from build123d import *

# Parameters (mm, degrees)
SKETCH1_R               = 27.1
SKETCH1_R_2             = 25.2
BOSS_EXTRUDE1_DEPTH     = 300
SKETCH2_R               = 2.9
CUT_EXTRUDE1_DEPTH      = 28.1
CUT_EXTRUDE1_DEPTH_BACK = 28.1


with BuildPart() as part:
    # Sketch1 → Boss-Extrude1 (new body)
    with BuildSketch(Plane(origin=(0, 0, 0), x_dir=(1, 0, 0), z_dir=(0, 1, 0))):
        Circle(SKETCH1_R)
        Circle(SKETCH1_R_2, mode=Mode.SUBTRACT)
    extrude(amount=BOSS_EXTRUDE1_DEPTH)

    # Sketch2 → Cut-Extrude1 (cut, two sides)
    with BuildSketch(Plane(origin=(0, 0, 0), x_dir=(0, 0, -1), z_dir=(1, 0, 0))) as cut_extrude1_sk:
        with Locations((0, 10)):
            Circle(SKETCH2_R)
        with Locations((0, 25.5)):
            Circle(SKETCH2_R)
    extrude(amount=CUT_EXTRUDE1_DEPTH, mode=Mode.SUBTRACT)
    extrude(cut_extrude1_sk.sketch, amount=-CUT_EXTRUDE1_DEPTH_BACK, mode=Mode.SUBTRACT)


solid = part.part
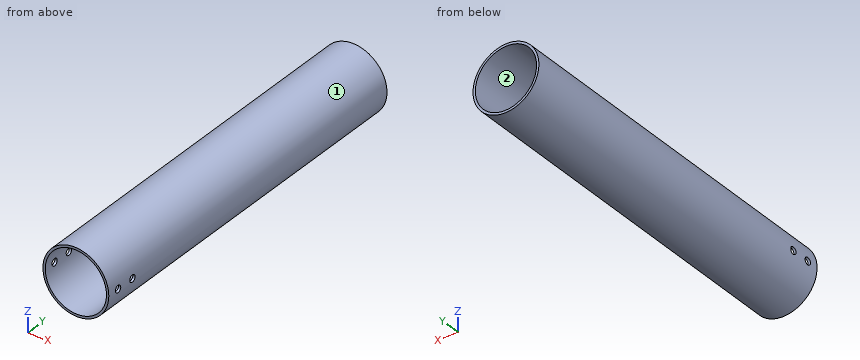
Geometry check sheet. Reference: the model listing, model coordinates, mm. Face numbers are marked on the shaded views. Coordinates: 2 decimals unless noted, no trailing zeros. Order: outer loops, then holes, each group sorted by start corner. A loop starts at its lowest first (then second) coordinate and runs counter-clockwise, first axis right, second up. Notation, with made-up numbers: (60.5, 46) - (86.5, 46) arc R11 ccw to (86.5, 59) - close; hole circle Ø9 at (37, 64). An arc over 180 degrees is marked (long way). Answer in a Markdown table with one row per item. Add a question column.
1) Cross-section at D-D, the plane y = 150.5. Record the cut outline in (x, z).
2) Material ranges on line 1 along Y through (x, z) = (-25.95, 0); line 2 along X through (y, z) = (81.5, 7); line 3 along X through (y, z) = (107, 22), recorded low to high. Write a range as [from, to].
3) Cross-section at C-C, the plane y = 10. Record the cut outline in (x, z), then the cut area to 3 significant figures.
4) Release check for a two-part mould opening along X. For the marked faces 1 and 2 record: +X half, -X half, draft (parallel to the pull), parting line (faces both ways), or undercut.
5) Cross-section at A-A, the plane z = 0. Record the cut outline in (x, y).
6) Gauge pin test, flat ends, axial feed: P1, Ø12, axis at x = -6.5, y = 168.5, coming from the -Z side; P2, Ø4, axis at y = 221, z = 5.5, coming from the +X side; P3, Ø5, axis at x = 20.5, y = 240.5, coming from the +Z side. Record the tip position at first contact, or that the pin passes through.
7) Cross-section at B-B, the plane x = 0. Record the cut outline in (y, z).
Check result:
| question | item | result |
|---|---|---|
| 1 | outline | circle Ø54.2 at (0, 0); hole circle Ø50.4 at (0, 0) |
| 2 | line 1 | y = [0, 7.1], [12.9, 22.6], [28.4, 300] |
| 2 | line 2 | x = [-26.18, -24.21], [24.21, 26.18] |
| 2 | line 3 | x = [-15.82, -12.29], [12.29, 15.82] |
| 3 | outline | (-26.94, -2.9) arc R27.1 ccw to (26.94, -2.9) - (25.03, -2.9) arc R25.2 cw to (-25.03, -2.9) - close; (-26.94, 2.9) - (-25.03, 2.9) arc R25.2 cw to (25.03, 2.9) - (26.94, 2.9) arc R27.1 ccw to start |
| 3 | area | 290 mm² |
| 4 | face 1 | parting line |
| 4 | face 2 | undercut |
| 5 | outline | (-27.1, 0) - (-25.2, 0) - (-25.2, 7.1) - (-27.1, 7.1) - close; (-27.1, 12.9) - (-25.2, 12.9) - (-25.2, 22.6) - (-27.1, 22.6) - close; (-27.1, 28.4) - (-25.2, 28.4) - (-25.2, 300) - (-27.1, 300) - close; (25.2, 0) - (27.1, 0) - (27.1, 7.1) - (25.2, 7.1) - close; (25.2, 12.9) - (27.1, 12.9) - (27.1, 22.6) - (25.2, 22.6) - close; (25.2, 28.4) - (27.1, 28.4) - (27.1, 300) - (25.2, 300) - close |
| 6 | P1 | stops at z = -27.1 |
| 6 | P2 | stops at x = 26.87 |
| 6 | P3 | stops at z = 20.26 |
| 7 | outline | (0, -27.1) - (300, -27.1) - (300, -25.2) - (0, -25.2) - close; (0, 25.2) - (300, 25.2) - (300, 27.1) - (0, 27.1) - close |
